Geometry: final body of the model. Coordinates: model frame, mm. A direction names the side the tool comes from. Give positions to 0.01 mm unless a question says otherwise; leave off trailing zeros. Write each loop counter-clockwise with the first axis right and the second up, starting at its lowest first coordinate (ties: lowest second). Pieces come first, ordered by that corner, then holes. Notation, with made-up numbers: M 54,80.5 L 65,80.5 A26 cw 65,110.5 Z; hole C 4,-7 d6. An arc over 180 degrees is marked long. Answer as a JSON object with one key per item and string values.
from build123d import *

# Parameters (mm, degrees)
F2_DEPTH     = 5.715
F3_R         = 5.08
F4_R         = 2.54
F0_R         = 10.16
F0_R_2       = 3.175
F5_DEPTH     = 5.715
F7_DEPTH     = 25.4
F9_DEPTH     = 5.715
F10_T1_DEPTH = 10.4031459942
F10_T3_DEPTH = 10.4031462213
F10_T5_DEPTH = 21.8251062119
F12_DEPTH    = 12.7
F13_R        = 0.508
F14_SIZE     = 2.54


# Not quite as in the source:
# - a fillet or chamfer that OpenCascade refuses, or shapes differently, is made with other operations: its cross-section is extruded or revolved along the edge and cut away or added


with BuildPart() as f2:
    # F1 (on Right) → F2 (new body, symmetric)
    with BuildSketch(Plane.YZ):
        Polygon((20.3924354673, 0.8880047341), (69.85, 4.8502287827), (76.2, 14.35636729), (12.8064267337, 14.35636729), (2.9200423986, 9.7313386741), (8.2383593544, 1.7451149179), (4.8682624474, -6.6303843632), (5.9557488763, -8.2313216024), align=None)
    extrude(amount=F2_DEPTH, both=True)

    # F3
    f3_edges = [f2.edges().sort_by_distance(p)[0] for p in [
        (0, 12.806427, 14.356367),
        (0, 69.85, 4.850229),
        (0, 20.392435, 0.888005),
    ]]
    fillet(f3_edges, radius=F3_R)

    # F4
    f4_edges = [f2.edges().sort_by_distance(p)[0] for p in [
        (0, 76.2, 14.356367),
    ]]
    fillet(f4_edges, radius=F4_R)

    # F0 (on Right) → F5 (join)
    with BuildSketch(Plane.YZ):
        Circle(F0_R)
        Circle(F0_R_2, mode=Mode.SUBTRACT)
    extrude(amount=F5_DEPTH)

    # F6 (on Right) → F7 (cut)
    with BuildSketch(Plane.YZ):
        with BuildLine():
            Line((19.0573167056, 0), (5.4165862694, 8.5957078351))
            ThreePointArc((5.4165862694, 8.5957078351), (-10.1595718617, -0.0932715764), (5.5734885208, -8.4948116935))
            Line((5.5734885208, -8.4948116935), (19.0573167056, 0))
        make_face()
    extrude(amount=-F7_DEPTH, mode=Mode.SUBTRACT)

    # F8 (on Right) → F9 (join, symmetric)
    with BuildSketch(Plane.YZ):
        with BuildLine():
            Line((0.5413664183, -10.9723807834), (0.5413664183, -10.1455666378))
            ThreePointArc((0.5413664183, -10.1455666378), (-6.0054239987, -8.1951499434), (-9.8373776994, -2.54))
            Line((-9.8373776994, -2.54), (-25.4, -2.54))
            Line((-25.4, -2.54), (-25.4, -6.360667292))
            Line((-25.4, -6.360667292), (-2.5253696451, -10.9723807834))
            Line((-2.5253696451, -10.9723807834), (0.5413664183, -10.9723807834))
        make_face()
    extrude(amount=F9_DEPTH, both=True)

    # F10: fillet of radius 2.54 on 2 edges, made by hand

    # F10_s2 → F10_t1 (cut)
    with BuildSketch(Plane.YZ.offset(-10.4031461077)):
        with BuildLine():
            ThreePointArc((0.5413664183, -10.1455666378), (-0.3091706163, -10.7565034211), (-1.3338920247, -10.9723807834))
            Line((-1.3338920247, -10.9723807834), (0.5413664183, -10.9723807834))
            Line((0.5413664183, -10.9723807834), (0.5413664183, -10.1455666378))
        make_face()
    extrude(amount=F10_T1_DEPTH, mode=Mode.SUBTRACT)

    # F10_s4 → F10_t3 (cut)
    with BuildSketch(Plane.YZ.offset(-1.135e-07)):
        with BuildLine():
            ThreePointArc((0.5413664183, -10.1455666378), (-0.3091706163, -10.7565034211), (-1.3338920247, -10.9723807834))
            Line((-1.3338920247, -10.9723807834), (0.5413664183, -10.9723807834))
            Line((0.5413664183, -10.9723807834), (0.5413664183, -10.1455666378))
        make_face()
    extrude(amount=F10_T3_DEPTH, mode=Mode.SUBTRACT)

    # F10_s6 → F10_t5 (cut)
    with BuildSketch(Plane.YZ.offset(-10.912553106)):
        with BuildLine():
            ThreePointArc((-25.4, -4.2816460496), (-24.8255331463, -5.8904591062), (-23.3619846843, -6.7715479306))
            Line((-23.3619846843, -6.7715479306), (-25.4, -6.360667292))
            Line((-25.4, -6.360667292), (-25.4, -4.2816460496))
        make_face()
    extrude(amount=F10_T5_DEPTH, mode=Mode.SUBTRACT)

    # F11 (on face) → F12 (join)
    with BuildSketch(Plane.XZ.offset(25.4)):
        Polygon((2.7630305849, -0.762), (2.032, -2.54), (5.715, -2.54), (5.715, -0.254), align=None)
        Polygon((-5.715, -2.54), (-2.032, -2.54), (-2.7630305849, -0.762), (-5.715, -0.254), align=None)
    extrude(amount=-F12_DEPTH)

    # F13
    f13_edges = [f2.edges().sort_by_distance(p)[0] for p in [
        (-2.763031, -19.05, -0.762),
        (2.763031, -19.05, -0.762),
    ]]
    fillet(f13_edges, radius=F13_R)

    # F14
    f14_edges = [f2.edges().sort_by_distance(p)[0] for p in [
        (5.715, -3.175, 0),
    ]]
    chamfer(f14_edges, length=F14_SIZE)


solid = f2.part
1) Contact query for flat-ended pins moving along their axis: P1, Ø1, axis at x = 3, z = -1.5, coming from the +Y side; P2, Ø1.1, axis at x = -3.5, z = -1, coming from the +Y side; P3, Ø5.5, axis at y = 0, z = 0, coming from the -X side; P4, Ø0.7, axis at x = 5, z = -1.5, coming from the +Y side. Output: stop coordinate, or through.
Geometry check:
{"P1": "stops at y = 17.4", "P2": "stops at y = -12.7", "P3": "passes through", "P4": "stops at y = 17.17"}
2) Set-up query: faces 1 (the flat face through (-2.82, 12.31, 4.25)), 2 (the cylindrical face through (0.08, 73.707, 12.98)), 3 (the flat face through (2.62, 12.551, -4.065)), 4 (the flat face through (4, -12.7, -2)), 5 (the flat face through (0, 4, 0)). Return all of +Z, -Z, +X, -X, +Y, -Y with unobstructed straight access to the full face (end or side cutting, diameter ignored); none if empty.
Geometry check:
{"face 1": "-Z, -X, -Y", "face 2": "+X, -X, +Y", "face 3": "-Z, +X, -X, +Y", "face 4": "+Z, +X, -X", "face 5": "-X"}
3) Cut plane B-B on y = 23.5. Return loops of the section in (x, z) (3 decimals), and give its area (3 significant figures).
Geometry check:
{"outline": "M -5.715,1.137 L 5.715,1.137 L 5.715,14.356 L -5.715,14.356 Z", "area": "151 mm2"}
4) Line query: line 1 (Z direction, x = -2.25, y = 46); line 2 (Z direction, x = 1.05, y = 0) (3 decimals); line 3 (X direction, y = 16, z = -1) (3 decimals). Output: solid intervals per line, ascending. Write a range as from..to.
Geometry check:
{"line 1": "z = 2.94..14.36", "line 2": "z = -10.594..-3.175, 3.175..10.16", "line 3": "x = 0..5.715"}
5) Pull-direction query (X, two-part tool) for faces 6 (the flat face through (5.715, 24, 4)), 7 (the flat face through (-5.715, -15, -6)), 8 (the cylindrical face through (-0.08, -24.84, -5.87)), 9 (the flat face through (-4.359, -19.139, -0.487)); classes: pulls with the +X half, pulls with the -X half, needs draft (parallel to the pull), parting line crosses it, or undercut.
Geometry check:
{"face 6": "pulls with the +X half", "face 7": "pulls with the -X half", "face 8": "needs draft", "face 9": "undercut"}
6) Cut plane A-A on y = 66.5. Return loops of the section in (x, z) (3 decimals), and give its area (3 significant figures).
Geometry check:
{"outline": "M -5.715,4.582 L 5.715,4.582 L 5.715,14.356 L -5.715,14.356 Z", "area": "112 mm2"}
